Source: CAD feature listing. Evaluate the final solid. Frame: model axes, mm. Round coordinates to 2 decimals unless told otherwise and drop trailing zeros. Loops run counter-clockwise (first coordinate to the right, second up) from the corner with the lowest first, then second, coordinate; pieces in that order, holes last. Notation, with made-up numbers: (10, 51) -> (18, 51) arc R30 ccw to (18, 83) -> close; hole circle Ø1 at (-8, 14.25). An arc over 180 degrees is marked (long way). Put each result on its own line as item: value. Start each with the question number.
1. Contact query for flat-ended pins moving along their axis: pin 1 (2 mm diameter, centred on y = 28.5, z = 4, fed in from -X); pin 2 (6 mm diameter, centred on x = -2, z = -4.5, fed in from +Y); pin 3 (3 mm diameter, centred on y = 5, z = 3, fed in from +X). Output: stop coordinate, or through.
2. Draft query along Y for faces 1 (the flat face through (0, 0, 0)), 2 (the cylindrical face through (1.73, 0.99, -7.81)), 3 (the conical face through (3.373, 4.944, -2.586)). Return one class per face: pulls with the +Y half, pulls with the -Y half, needs draft (parallel to the pull), parting line crosses it, or undercut.
3. Material intervals for L1, parallel to Y at x = 0.25, z = -6; L2, parallel to Y at x = 5, z = -0.25; L3, parallel to X at y = 6.5, z = -0.25, sorted ascending.
4. Cut plane B-B (x = -5.5). State how many separate pieces and enclosed holes the cut face has, then the cut area to 3 significant figures.
5. Cut plane D-D (y = 18.5). Return the cut outline in (x, z), then the cut area to 3 significant figures.
6. Cut plane A-A (y = 8.5). Return the cut outline in (x, z), then the cut area to 3 significant figures.
```python
from build123d import *


with BuildPart() as f1:
    # F0 (on Top) → F1 (revolve)
    with BuildSketch(Plane.XY):
        with BuildLine():
            Line((-8, 0), (0, 0))
            Line((0, 0), (0, 37.344937))
            ThreePointArc((0, 37.344937), (-6.387622, 32.375548), (-3.141686, 24.962018))
            ThreePointArc((-3.141686, 24.962018), (-3.436771, 17.048593), (-6.78, 9.87))
            Line((-6.78, 9.87), (-6.78, 6.87))
            Line((-6.78, 6.87), (-4, 5.14))
            Line((-4, 5.14), (-8, 2))
            Line((-8, 2), (-8, 0))
        make_face()
    revolve(axis=Axis((0, 18.672468, 0), (0, 1, 0)))


solid = f1.part
```
Solution:
1. pin 1: stops at x = -5.53
1. pin 2: stops at y = 37.06
1. pin 3: stops at x = 5.52
2. face 1: pulls with the -Y half
2. face 2: needs draft
2. face 3: undercut
3. L1: y = 0 to 3.57, 6.39 to 11, 28.04 to 33.47
3. L2: y = 0 to 4.35, 5.77 to 12.76, 26.47 to 35.04
3. L3: x = -6.18 to 6.18
4. separate pieces: 3
4. enclosed holes: 0
4. area: 117 mm^2
5. outline: circle Ø6.29 at (0, 0)
5. area: 31.0 mm^2
6. outline: circle Ø13.56 at (0, 0)
6. area: 144 mm^2
